Build history of the part. All positions in model axes, mm. Face numbers are marked on the shaded views. A direction names the side the tool comes from. Give positions to 0.01 mm unless a question says otherwise; leave off trailing zeros. Order: outer loops, then holes, each group sorted by start corner. A loop starts at its lowest first (then second) coordinate and runs counter-clockwise, first axis right, second up. Notation, with made-up numbers: (8.25, 73.25) -> (54.25, 73.25) arc R24 cw to (54.25, 106.25) -> close; hole circle Ø11 at (87, 79). An arc over 180 degrees is marked (long way). One line per item, written item: value. Start each with the question number.
(1) Probe line 1 (Z direction, x = 127.5, y = 34.35); line 2 (X direction, y = 35, z = -5); line 3 (Y direction, x = 22, z = -45.5). List the from-to ranges inside material, lowest first.
(2) Which spindle directions (+Z, -Z, +X, -X, +Y, -Y) get a long thin tool onto all of the face, cutting with end or side? Do the marked faces 1, 2 and 3. Say none if no direction does.
(3) Saw through at D-D on x = 47. Give the cut face in (y, z).
(4) Saw through at C-C on y = 29.5. Count the separate pieces of the cut face and the enclosed holes in it, plus the area to 3 significant figures.
(5) Two-plate mould, pull along Z, no slides. Class the marked faces 4 and 5: +Z half, -Z half, draft (parallel to the pull), parting line (faces both ways), or undercut.
(6) Pin check, flat tips, straight feed: pin 1 (1.4 mm diameter, centred on x = 37, z = -2, fed in from +Y); pin 2 (0.5 mm diameter, centred on y = 28, z = -111, fed in from +X); pin 3 (1.2 mm diameter, centred on y = 35, z = -6, fed in from +X). Stop position of each tip, or through.
(7) Saw through at A-A on x = 19. Give the cut face in (y, z).
(8) Saw through at B-B on z = -81.5. Give the cut face in (x, y), plus the area to 3 significant figures.
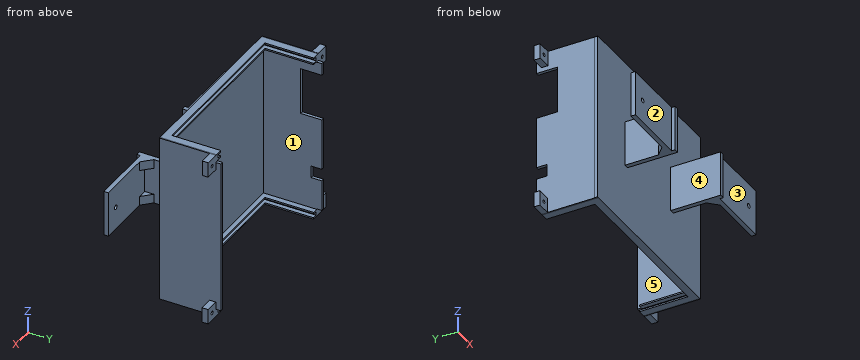
```python
from build123d import *

# Parameters (mm, degrees)
SKETCH1_W            = 124.4
SKETCH1_H            = 111.7
BOSS_EXTRUDE1_DEPTH  = 2
SKETCH2_W            = 2
SKETCH2_H            = 101.7
BOSS_EXTRUDE2_DEPTH  = 38.5
SKETCH3_W            = 121.7
SKETCH3_H            = 4.7
BOSS_EXTRUDE3_DEPTH  = 3
SKETCH5_W            = 116.3
SKETCH5_H            = 2.7
CUT_EXTRUDE8_DEPTH   = 3
SKETCH14_W           = 121.7
SKETCH14_H           = 4.7
BOSS_EXTRUDE6_DEPTH  = 3
SKETCH15_W           = 116.3
SKETCH15_H           = 2.7
CUT_EXTRUDE14_DEPTH  = 3
SKETCH18_W           = 2
SKETCH18_H           = 0.3
BOSS_EXTRUDE7_DEPTH  = 35.2
SKETCH19_W           = 5.7
SKETCH19_H           = 4.7
BOSS_EXTRUDE8_DEPTH  = 32.2
SKETCH20_W           = 2.7
SKETCH20_H           = 32.2
CUT_EXTRUDE15_DEPTH  = 3
SKETCH21_W           = 2.7
SKETCH21_H           = 32.2
CUT_EXTRUDE16_DEPTH  = 3
SKETCH24_W           = 2.7
SKETCH24_H           = 32.2
CUT_EXTRUDE18_DEPTH  = 3
SKETCH25_W           = 2.7
SKETCH25_H           = 32.2
CUT_EXTRUDE19_DEPTH  = 3
SKETCH30_W           = 31
SKETCH30_H           = 14
SKETCH30_W_2         = 8
SKETCH30_H_2         = 7
CUT_EXTRUDE23_DEPTH  = 2
SKETCH31_W           = 6
SKETCH31_H           = 36.2
BOSS_EXTRUDE9_DEPTH  = 1.35
FILLET1_R            = 2
SKETCH33_W           = 99.7
SKETCH33_H           = 3
BOSS_EXTRUDE11_DEPTH = 1.35
SKETCH43_W           = 1.229805297
SKETCH43_H           = 112.077966817
CUT_EXTRUDE25_DEPTH  = 38.2
SKETCH47_W           = 57.12
SKETCH47_H           = 30
BOSS_EXTRUDE22_DEPTH = 38
SKETCH49_W           = 51.12
SKETCH49_H           = 30
CUT_EXTRUDE30_DEPTH  = 38
SKETCH51_W           = 2.352063359
SKETCH51_H           = 112.382279656
CUT_EXTRUDE33_DEPTH  = 77.2
SKETCH54_W           = 10
SKETCH54_H           = 4.16571725
SKETCH54_H_2         = 4.016594053
BOSS_EXTRUDE23_DEPTH = 9
SKETCH55_W           = 10
SKETCH55_H           = 3.950767522
SKETCH55_W_2         = 9.95127899
SKETCH55_H_2         = 4
BOSS_EXTRUDE24_DEPTH = 9
SKETCH56_R           = 1.1
CUT_EXTRUDE34_DEPTH  = 10
SKETCH57_R           = 1
CUT_EXTRUDE35_DEPTH  = 99.41
SKETCH58_W           = 30
SKETCH58_H           = 3
BOSS_EXTRUDE25_DEPTH = 43
SKETCH59_W           = 30
SKETCH59_H           = 3.021561104
BOSS_EXTRUDE26_DEPTH = 43
BOSS_EXTRUDE28_DEPTH = 6
BOSS_EXTRUDE29_DEPTH = 6
BOSS_EXTRUDE30_DEPTH = 6
BOSS_EXTRUDE31_DEPTH = 6
SKETCH64_W           = 30
SKETCH64_H           = 6.546083461
CUT_EXTRUDE36_DEPTH  = 101.12
SKETCH65_R           = 1.5
CUT_EXTRUDE37_DEPTH  = 6
SKETCH67_R           = 1.5
CUT_EXTRUDE39_DEPTH  = 6


with BuildPart() as part:
    # Sketch1 → Boss-Extrude1 (new body)
    with BuildSketch(Plane(origin=(0, 0, 0), x_dir=(1, 0, 0), z_dir=(0, 1, 0))):
        with Locations((62.2, 55.85)):
            Rectangle(SKETCH1_W, SKETCH1_H)
    extrude(amount=BOSS_EXTRUDE1_DEPTH)

    # Sketch2 → Boss-Extrude2 (add)
    with BuildSketch(Plane(origin=(0, 2, 0), x_dir=(1, 0, 0), z_dir=(0, 1, 0))):
        with Locations((122.05, 55.85)):
            Rectangle(SKETCH2_W, SKETCH2_H)
        with Locations((2.35, 55.85)):
            Rectangle(SKETCH2_W, SKETCH2_H)
    extrude(amount=BOSS_EXTRUDE2_DEPTH)

    # Sketch3 → Boss-Extrude3 (add)
    with BuildSketch(Plane(origin=(0, 2, 0), x_dir=(1, 0, 0), z_dir=(0, 1, 0))):
        with Locations((62.2, 2.35)):
            Rectangle(SKETCH3_W, SKETCH3_H)
    extrude(amount=BOSS_EXTRUDE3_DEPTH)

    # Sketch5 → Cut-Extrude8 (cut)
    with BuildSketch(Plane(origin=(0, 5, 0), x_dir=(1, 0, 0), z_dir=(0, 1, 0))):
        with Locations((62.2, 2.35)):
            Rectangle(SKETCH5_W, SKETCH5_H)
    extrude(amount=-CUT_EXTRUDE8_DEPTH, mode=Mode.SUBTRACT)

    # Sketch14 → Boss-Extrude6 (add)
    with BuildSketch(Plane(origin=(0, 2, 0), x_dir=(1, 0, 0), z_dir=(0, 1, 0))):
        with Locations((62.2, 109.35)):
            Rectangle(SKETCH14_W, SKETCH14_H)
    extrude(amount=BOSS_EXTRUDE6_DEPTH)

    # Sketch15 → Cut-Extrude14 (cut)
    with BuildSketch(Plane(origin=(0, 5, 0), x_dir=(1, 0, 0), z_dir=(0, 1, 0))):
        with Locations((62.2, 109.35)):
            Rectangle(SKETCH15_W, SKETCH15_H)
    extrude(amount=-CUT_EXTRUDE14_DEPTH, mode=Mode.SUBTRACT)

    # Sketch18 → Boss-Extrude7 (add)
    with BuildSketch(Plane(origin=(0, 2, 0), x_dir=(1, 0, 0), z_dir=(0, 1, 0))):
        with Locations((2.35, 106.85)):
            Rectangle(SKETCH18_W, SKETCH18_H)
        with Locations((122.05, 106.85)):
            Rectangle(SKETCH18_W, SKETCH18_H)
        with Locations((122.05, 4.85)):
            Rectangle(SKETCH18_W, SKETCH18_H)
        with Locations((2.35, 4.85)):
            Rectangle(SKETCH18_W, SKETCH18_H)
    extrude(amount=BOSS_EXTRUDE7_DEPTH)

    # Sketch19 → Boss-Extrude8 (add)
    with BuildSketch(Plane(origin=(0, 5, 0), x_dir=(1, 0, 0), z_dir=(0, 1, 0))):
        with Locations((120.2, 2.35)):
            Rectangle(SKETCH19_W, SKETCH19_H)
        with Locations((4.2, 2.35)):
            Rectangle(SKETCH19_W, SKETCH19_H)
        with Locations((120.2, 109.35)):
            Rectangle(SKETCH19_W, SKETCH19_H)
        with Locations((4.2, 109.35)):
            Rectangle(SKETCH19_W, SKETCH19_H)
    extrude(amount=BOSS_EXTRUDE8_DEPTH)

    # Sketch20 → Cut-Extrude15 (cut)
    with BuildSketch(Plane.ZY.offset(-117.35)):
        with Locations((-109.35, 21.1)):
            Rectangle(SKETCH20_W, SKETCH20_H)
    extrude(amount=-CUT_EXTRUDE15_DEPTH, mode=Mode.SUBTRACT)

    # Sketch21 → Cut-Extrude16 (cut)
    with BuildSketch(Plane(origin=(7.05, 0, 0), x_dir=(0, 0, -1), z_dir=(1, 0, 0))):
        with Locations((109.35, 21.1)):
            Rectangle(SKETCH21_W, SKETCH21_H)
    extrude(amount=-CUT_EXTRUDE16_DEPTH, mode=Mode.SUBTRACT)

    # Sketch24 → Cut-Extrude18 (cut)
    with BuildSketch(Plane(origin=(7.05, 0, 0), x_dir=(0, 0, -1), z_dir=(1, 0, 0))):
        with Locations((2.35, 21.1)):
            Rectangle(SKETCH24_W, SKETCH24_H)
    extrude(amount=-CUT_EXTRUDE18_DEPTH, mode=Mode.SUBTRACT)

    # Sketch25 → Cut-Extrude19 (cut)
    with BuildSketch(Plane.ZY.offset(-117.35)):
        with Locations((-2.35, 21.1)):
            Rectangle(SKETCH25_W, SKETCH25_H)
    extrude(amount=-CUT_EXTRUDE19_DEPTH, mode=Mode.SUBTRACT)

    # Sketch30 → Cut-Extrude23 (cut)
    with BuildSketch(Plane.ZY.offset(-1.35)):
        with Locations((-28.5, 33.5)):
            Rectangle(SKETCH30_W, SKETCH30_H)
        with Locations((-82.2, 37)):
            Rectangle(SKETCH30_W_2, SKETCH30_H_2)
    extrude(amount=-CUT_EXTRUDE23_DEPTH, mode=Mode.SUBTRACT)

    # Sketch31 → Boss-Extrude9 (add)
    with BuildSketch(Plane(origin=(123.05, 0, 0), x_dir=(0, 0, -1), z_dir=(1, 0, 0))):
        with Locations((3, 20.1)):
            Rectangle(SKETCH31_W, SKETCH31_H)
        with Locations((108.7, 20.1)):
            Rectangle(SKETCH31_W, SKETCH31_H)
    extrude(amount=BOSS_EXTRUDE9_DEPTH)

    # Fillet1
    fillet1_edges = [part.edges().sort_by_distance(p)[0] for p in [
        (0, 1, 0),
        (124.4, 19.1, 0),
        (124.4, 19.1, -111.7),
        (0, 1, -111.7),
    ]]
    fillet(fillet1_edges, radius=FILLET1_R)

    # Sketch33 → Boss-Extrude11 (add)
    with BuildSketch(Plane(origin=(123.05, 0, 0), x_dir=(0, 0, -1), z_dir=(1, 0, 0))):
        with Locations((55.85, 3.5)):
            Rectangle(SKETCH33_W, SKETCH33_H)
    extrude(amount=BOSS_EXTRUDE11_DEPTH)

    # Sketch43 → Cut-Extrude25 (cut, through all)
    with BuildSketch(Plane(origin=(0, 37.2, 0), x_dir=(1, 0, 0), z_dir=(0, 1, 0))):
        with Locations((0.614902649, 56.193231497)):
            Rectangle(SKETCH43_W, SKETCH43_H)
    extrude(amount=-CUT_EXTRUDE25_DEPTH, mode=Mode.SUBTRACT)

    # Sketch47 → Boss-Extrude22 (add)
    with BuildSketch(Plane(origin=(0, 0, 0), x_dir=(-1, 0, 0), z_dir=(0, -1, 0))):
        with Locations((-62.2, 55.85)):
            Rectangle(SKETCH47_W, SKETCH47_H)
    extrude(amount=BOSS_EXTRUDE22_DEPTH)

    # Sketch49 → Cut-Extrude30 (cut)
    with BuildSketch(Plane(origin=(0, -38, 0), x_dir=(-1, 0, 0), z_dir=(0, -1, 0))):
        with Locations((-62.2, 55.85)):
            Rectangle(SKETCH49_W, SKETCH49_H)
    extrude(amount=-CUT_EXTRUDE30_DEPTH, mode=Mode.SUBTRACT)

    # Sketch51 → Cut-Extrude33 (cut, through all)
    with BuildSketch(Plane(origin=(0, 38.2, 0), x_dir=(1, 0, 0), z_dir=(0, 1, 0))):
        with Locations((124.22603168, 56.299711796)):
            Rectangle(SKETCH51_W, SKETCH51_H)
    extrude(amount=-CUT_EXTRUDE33_DEPTH, mode=Mode.SUBTRACT)

    # Sketch54 → Boss-Extrude23 (add)
    with BuildSketch(Plane.ZY.offset(-1.35)):
        with Locations((-5, 35.117141375)):
            Rectangle(SKETCH54_W, SKETCH54_H)
        with Locations((-106.7, 35.191702973)):
            Rectangle(SKETCH54_W, SKETCH54_H_2)
    extrude(amount=BOSS_EXTRUDE23_DEPTH)

    # Sketch55 → Boss-Extrude24 (add)
    with BuildSketch(Plane(origin=(123.05, 0, 0), x_dir=(0, 0, -1), z_dir=(1, 0, 0))):
        with Locations((5, 35.224616239)):
            Rectangle(SKETCH55_W, SKETCH55_H)
        with Locations((106.724360505, 35.2)):
            Rectangle(SKETCH55_W_2, SKETCH55_H_2)
    extrude(amount=BOSS_EXTRUDE24_DEPTH)

    # Sketch56 → Cut-Extrude34 (cut)
    with BuildSketch(Plane(origin=(0, 37.2, 0), x_dir=(1, 0, 0), z_dir=(0, 1, 0))):
        with Locations((-3.1, 106.7)):
            Circle(SKETCH56_R)
        with Locations((127.5, 106.7)):
            Circle(SKETCH56_R)
        with Locations((127.5, 5)):
            Circle(SKETCH56_R)
        with Locations((-3.1, 5)):
            Circle(SKETCH56_R)
    extrude(amount=-CUT_EXTRUDE34_DEPTH, mode=Mode.SUBTRACT)

    # Sketch57 → Cut-Extrude35 (cut, through all)
    with BuildSketch(Plane(origin=(90.76, 0, 0), x_dir=(0, 0, -1), z_dir=(1, 0, 0))):
        with Locations((45.85, -34)):
            Circle(SKETCH57_R)
        with Locations((65.85, -34)):
            Circle(SKETCH57_R)
    extrude(amount=-CUT_EXTRUDE35_DEPTH, mode=Mode.SUBTRACT)

    # Sketch58 → Boss-Extrude25 (add)
    with BuildSketch(Plane(origin=(90.76, 0, 0), x_dir=(0, 0, -1), z_dir=(1, 0, 0))):
        with Locations((55.85, -29.25)):
            Rectangle(SKETCH58_W, SKETCH58_H)
    extrude(amount=BOSS_EXTRUDE25_DEPTH)

    # Sketch59 → Boss-Extrude26 (add)
    with BuildSketch(Plane.ZY.offset(-33.64)):
        with Locations((-55.85, -29.239219448)):
            Rectangle(SKETCH59_W, SKETCH59_H)
    extrude(amount=BOSS_EXTRUDE26_DEPTH)

    # Sketch61 → Boss-Extrude28 (add)
    with BuildSketch(Plane.XY.offset(-40.85)):
        Polygon((90.76, -21.75), (96.76, -27.75), (90.76, -27.75), align=None)
    extrude(amount=-BOSS_EXTRUDE28_DEPTH)

    # Sketch62 → Boss-Extrude29 (add)
    with BuildSketch(Plane(origin=(0, 0, -70.85), x_dir=(-1, 0, 0), z_dir=(0, 0, -1))):
        Polygon((-90.76, -21.75), (-90.76, -27.75), (-96.76, -27.75), align=None)
    extrude(amount=-BOSS_EXTRUDE29_DEPTH)

    # Sketch60 → Boss-Extrude30 (add)
    with BuildSketch(Plane.XY.offset(-40.85)):
        Polygon((27.64, -27.728438896), (33.64, -21.728438896), (33.64, -27.728438896), align=None)
    extrude(amount=-BOSS_EXTRUDE30_DEPTH)

    # Sketch63 → Boss-Extrude31 (add)
    with BuildSketch(Plane(origin=(0, 0, -70.85), x_dir=(-1, 0, 0), z_dir=(0, 0, -1))):
        Polygon((-33.64, -22.069435851), (-33.64, -27.728438896), (-27.64, -27.728438896), align=None)
    extrude(amount=-BOSS_EXTRUDE31_DEPTH)

    # Sketch64 → Cut-Extrude36 (cut, through all)
    with BuildSketch(Plane.ZY.offset(-33.64)):
        with Locations((-55.85, -36.27304173)):
            Rectangle(SKETCH64_W, SKETCH64_H)
    extrude(amount=-CUT_EXTRUDE36_DEPTH, mode=Mode.SUBTRACT)

    # Sketch65 → Cut-Extrude37 (cut)
    with BuildSketch(Plane(origin=(0, -30.75, 0), x_dir=(-1, 0, 0), z_dir=(0, -1, 0))):
        with Locations((-125.11, 55.85)):
            Circle(SKETCH65_R)
    extrude(amount=-CUT_EXTRUDE37_DEPTH, mode=Mode.SUBTRACT)

    # Sketch67 → Cut-Extrude39 (cut)
    with BuildSketch(Plane.XZ.offset(30.75)):
        with Locations((-0.71, -55.85)):
            Circle(SKETCH67_R)
    extrude(amount=-CUT_EXTRUDE39_DEPTH, mode=Mode.SUBTRACT)


solid = part.part
```
Results below:
1. line 1: z = -111.7 to -107.8, -105.6 to -101.75, -10 to -6.1, -3.9 to 0
1. line 2: x = -7.65 to -4.2, -2 to 3.35, 121.05 to 126.4, 128.6 to 132.05
1. line 3: y = -30.75 to -27.73, 0 to 2
2. face 1: +Y
2. face 2: +Z, -Z, -X, -Y
2. face 3: +Z, -Z, +X, -Y
3. outline: (0, -111.7) -> (5, -111.7) -> (5, -110.7) -> (2, -110.7) -> (2, -108) -> (5, -108) -> (5, -107) -> (2, -107) -> (2, -4.7) -> (5, -4.7) -> (5, -3.7) -> (2, -3.7) -> (2, -1) -> (5, -1) -> (5, 0) -> (0, 0) -> close
4. separate pieces: 3
4. enclosed holes: 0
4. area: 422 mm²
5. face 4: draft
5. face 5: undercut
6. pin 1: stops at y = 2
6. pin 2: stops at x = 123.05
6. pin 3: stops at x = 132.05
7. outline: (-30.75, -70.85) -> (-27.73, -70.85) -> (-27.73, -40.85) -> (-30.75, -40.85) -> close; (0, -111.7) -> (5, -111.7) -> (5, -110.7) -> (2, -110.7) -> (2, -108) -> (5, -108) -> (5, -107) -> (2, -107) -> (2, -4.7) -> (5, -4.7) -> (5, -3.7) -> (2, -3.7) -> (2, -1) -> (5, -1) -> (5, 0) -> (0, 0) -> close
8. outline: (1.23, 0) -> (123.05, 0) -> (123.05, 40.5) -> (121.05, 40.5) -> (121.05, 2) -> (3.35, 2) -> (3.35, 33.5) -> (1.35, 33.5) -> (1.35, 2) -> (1.23, 2) -> close
8. area: 384 mm²
